from build123d import *

# Parameters (mm, degrees)
PAD_DEPTH    = 0.5
PAD001_DEPTH = 1
SKETCH001_R  = 1
POCKET_DEPTH = 0.5


with BuildPart() as part:
    # Sketch (on DatumPlane) → Pad (new body)
    with BuildSketch(Plane.XY.offset(0.51)):
        with BuildLine():
            Line((-3.175, 3.175), (21.225, 3.175))
            ThreePointArc((22.225, 2.175), (21.932107, 2.882107), (21.225, 3.175))
            Line((22.225, 2.175), (22.225, -21.225))
            ThreePointArc((21.225, -22.225), (21.932107, -21.932107), (22.225, -21.225))
            Line((21.225, -22.225), (-2.175, -22.225))
            ThreePointArc((-3.175, -21.225), (-2.882107, -21.932107), (-2.175, -22.225))
            Line((-3.175, -21.225), (-3.175, 3.175))
        make_face()
    extrude(amount=PAD_DEPTH)

    # Sketch002 (on DatumPlane) → Pad001 (join)
    with BuildSketch(Plane.XY.offset(0.51)):
        with BuildLine():
            Line((-1.225, 0.725), (-1.225, -19.775))
            ThreePointArc((-1.225, -19.775), (-1.078553, -20.128553), (-0.725, -20.275))
            Line((-0.725, -20.275), (19.775, -20.275))
            ThreePointArc((19.775, -20.275), (20.128553, -20.128553), (20.275, -19.775))
            Line((20.275, -19.775), (20.275, 0.725))
            ThreePointArc((20.275, 0.725), (20.128553, 1.078553), (19.775, 1.225))
            Line((19.775, 1.225), (-0.725, 1.225))
            ThreePointArc((-0.725, 1.225), (-1.078553, 1.078553), (-1.225, 0.725))
        make_face()
    extrude(amount=PAD001_DEPTH)

    # Sketch001 (on DatumPlane) → Pocket (cut)
    with BuildSketch(Plane.XY.offset(0.51)):
        Circle(SKETCH001_R)
        with Locations((0, -19.05)):
            Circle(SKETCH001_R)
        with Locations((0, -9.525)):
            Circle(SKETCH001_R)
        with Locations((19.05, -19.05)):
            Circle(SKETCH001_R)
        with Locations((19.05, 0)):
            Circle(SKETCH001_R)
    extrude(amount=POCKET_DEPTH, mode=Mode.SUBTRACT)


solid = part.part
The model under review builds one solid part; all positions refer to its coordinate system, in mm. A direction names the side the tool comes from. Coordinates: 2 decimals unless noted, no trailing zeros. Loops run counter-clockwise (first coordinate to the right, second up) from the corner with the lowest first, then second, coordinate; pieces in that order, holes last.
(1) Wall thickness on L1, parallel to Y at x = 19.05, z = 0.8 (3 decimals); L2, parallel to Y at x = 0, z = 0.7 (3 decimals); L3, parallel to Y at x = 17, z = 1.1 (3 decimals): over which ranges is each line inside the solid? List them lowest first.
Determined:
L1: y = -22.225 to -20.05, -18.05 to -1, 1 to 3.175
L2: y = -22.225 to -20.05, -18.05 to -10.525, -8.525 to -1, 1 to 3.175
L3: y = -20.275 to 1.225
(2) Insertion check: P1, Ø2, axis at x = 19, y = 0, coming from the -Z side; P2, Ø0.6, axis at x = 0, y = 0, coming from the -Z side; P3, Ø0.6, axis at x = 13, z = 1.5, coming from the +Y side (3 decimals). Each pin has a flat end and moves straight along its axis. Give the tip position at first contact, or say it passes through.
Determined:
P1: stops at z = 0.51
P2: stops at z = 1.01
P3: stops at y = 1.225
(3) Draft analysis for pull direction X (two halves, no side actions). For faces 4 (the flat face through (9, -9, 1.51)), 5 (the flat face through (19, -19, 1.01)), 6 (the cylindrical face through (21.924, -21.94, 0.756)), state which applies: +X half, -X half, draft (parallel to the pull), parting line (faces both ways), or undercut.
Determined:
face 4: draft
face 5: undercut
face 6: +X half
(4) Consider section D-D, the plane x = 12.25. Give the boundary of the cut face in (y, z) (3 decimals).
Determined:
outline: (-22.225, 0.51) - (3.175, 0.51) - (3.175, 1.01) - (1.225, 1.01) - (1.225, 1.51) - (-20.275, 1.51) - (-20.275, 1.01) - (-22.225, 1.01) - close
(5) Tool access review of faces 1 (the flat face through (0, 0, 1.01)), 2 (the flat face through (-2, -9, 1.01)), 3 (the flat face through (9, -9, 0.51)): name each direction out of +Z, -Z, +X, -X, +Y, -Y from which nothing blocks a thin tool from reaching the whole face with its end or side.
Determined:
face 1: -Z
face 2: +Z
face 3: -Z, +X, -X, +Y, -Y
(6) Consider section A-A, the plane x = 19.05. Give the boundary of the cut face in (y, z) (3 decimals).
Determined:
outline: (-22.225, 0.51) - (-20.05, 0.51) - (-20.05, 1.01) - (-18.05, 1.01) - (-18.05, 0.51) - (-1, 0.51) - (-1, 1.01) - (1, 1.01) - (1, 0.51) - (3.175, 0.51) - (3.175, 1.01) - (1.225, 1.01) - (1.225, 1.51) - (-20.275, 1.51) - (-20.275, 1.01) - (-22.225, 1.01) - close
(7) Consider section B-B, the plane z = 0.8. Give the boundary of the cut face in (x, y) (3 decimals).
Determined:
outline: (-3.175, -21.225) arc R1 ccw to (-2.175, -22.225) - (21.225, -22.225) arc R1 ccw to (22.225, -21.225) - (22.225, 2.175) arc R1 ccw to (21.225, 3.175) - (-3.175, 3.175) - close; hole circle Ø2 at (0, -19.05); hole circle Ø2 at (0, -9.525); hole circle Ø2 at (0, 0); hole circle Ø2 at (19.05, -19.05); hole circle Ø2 at (19.05, 0)
(8) Consider section C-C, the plane y = -13.5. Give the boundary of the cut face in (x, z) (3 decimals).
Determined:
outline: (-3.175, 0.51) - (22.225, 0.51) - (22.225, 1.01) - (20.275, 1.01) - (20.275, 1.51) - (-1.225, 1.51) - (-1.225, 1.01) - (-3.175, 1.01) - close
